The model under review builds one solid part; all positions refer to its coordinate system, in mm. A direction names the side the tool comes from. Round coordinates to 2 decimals unless told otherwise and drop trailing zeros. Order: outer loops, then holes, each group sorted by start corner. A loop starts at its lowest first (then second) coordinate and runs counter-clockwise, first axis right, second up. Notation, with made-up numbers: M 77.5,4 L 134.5,4 A8 ccw 134.5,12 Z; hole C 11,41 d4. An arc over 180 degrees is marked long. Answer as a JSON object with one key per item and string values. Group by question number.
1) The part is to be moulded in two halves that separate along X. For faces 5 (the cylindrical face through (58, 1.61, -96.59)), 6 (the flat face through (-12.7, 2, -57)), 7 (the flat face through (63.5, 2, -95)), 8 (the flat face through (57, 2, -50.8)), say which applies: +X half, -X half, draft (parallel to the pull), parting line (faces both ways), or undercut.
2) Consider section D-D, the plane y = 2.2. Count the separate pieces of the cut face and the enclosed holes in it, then the cut area to 3 significant figures.
3) Consider section B-B, the plane z = -95.25. Write out the cut boundary in (x, y) (1 decimal), then the cut area to 3 significant figures.
4) Insertion check: pin 1 Ø1.6 at (y, z) = (1.5, -77) entering from -X; pin 2 Ø1.6 at (x, y) = (55.5, 1.5) entering from +Z; pin 3 Ø1 at (y, z) = (1.5, -22.5) entering from -X (3 decimals); pin 4 Ø1.9 at (x, z) = (57.15, -95.25) entering from +Y. Each pin has a flat end and moves straight along its axis. Give the tip position at first contact, or say it passes through.
5) Consider section A-A, the plane x = 57.15. Write out the cut boundary in (y, z) (1 decimal).
6) For faces 1 (the flat face through (50.8, 2, -77)), 2 (the flat face through (0, 2, -77)), 3 (the cylindrical face through (2.86, 1.57, -51.71)), 4 (the flat face through (0, 2, -124)), list the 3-axis set-ups (+Z, -Z, +X, -X, +Y, -Y) from which the entire face can be reached by the end or side of a thin tool; tool diameter is ignored.
7) Consider section C-C, the plane z = -57.15. Write out the cut boundary in (x, y) (1 decimal).
8) To check wall thickness, follow line 1 (Z direction, x = 57.15, y = 2.25); line 2 (X direction, y = 1.2, z = -95.25); line 3 (Z direction, x = 53.5, y = 1.7). State the ranges of each line that lie inside material, in increasing order.
```python
from build123d import *

# Parameters (mm, degrees)
SKETCH1_W           = 50.8
SKETCH1_H           = 76.2
BOSS_EXTRUDE1_DEPTH = 3.175
SKETCH2_W           = 18.415
SKETCH2_H           = 63.5
CUT_EXTRUDE1_DEPTH  = 3.175
SKETCH3_W           = 12.7
SKETCH3_H           = 12.7
SKETCH3_R           = 1.5875
BOSS_EXTRUDE2_DEPTH = 3.175
SKETCH7_W           = 50.8
SKETCH7_H           = 12.7
BOSS_EXTRUDE3_DEPTH = 3.175
SKETCH8_W           = 50.8
SKETCH8_H           = 57.15
BOSS_EXTRUDE4_DEPTH = 3.175
LPATTERN1_COUNT     = 2
LPATTERN1_PITCH     = 38.1
FILLET1_R           = 8.89
SKETCH9_W           = 6.35
SKETCH9_H           = 6.35
CUT_EXTRUDE2_DEPTH  = 3.175
SKETCH10_W          = 3.81
SKETCH10_H          = 50.8
CUT_EXTRUDE3_DEPTH  = 3.175
FILLET2_R           = 3.175
FILLET3_R           = 1.27


with BuildPart() as part:
    # Sketch1 → Boss-Extrude1 (new body)
    with BuildSketch(Plane(origin=(0, 0, 0), x_dir=(1, 0, 0), z_dir=(0, 1, 0))):
        with Locations((25.4, 38.1)):
            Rectangle(SKETCH1_W, SKETCH1_H)
    extrude(amount=BOSS_EXTRUDE1_DEPTH)

    # Sketch2 → Cut-Extrude1 (cut)
    with BuildSketch(Plane(origin=(0, 3.175, 0), x_dir=(1, 0, 0), z_dir=(0, 1, 0))):
        with Locations((13.0175, 31.75)):
            Rectangle(SKETCH2_W, SKETCH2_H)
        with Locations((37.7825, 31.75)):
            Rectangle(SKETCH2_W, SKETCH2_H)
    extrude(amount=-CUT_EXTRUDE1_DEPTH, mode=Mode.SUBTRACT)

    # Sketch3 → Boss-Extrude2 (add)
    with BuildSketch(Plane(origin=(0, 3.175, 0), x_dir=(1, 0, 0), z_dir=(0, 1, 0))):
        with Locations((-6.35, 57.15)):
            Rectangle(SKETCH3_W, SKETCH3_H)
        with Locations((-6.35, 57.15)):
            Circle(SKETCH3_R, mode=Mode.SUBTRACT)
        with Locations((57.15, 57.15)):
            Rectangle(SKETCH3_W, SKETCH3_H)
        with Locations((57.15, 57.15)):
            Circle(SKETCH3_R, mode=Mode.SUBTRACT)
    boss_extrude2 = extrude(amount=-BOSS_EXTRUDE2_DEPTH)

    # Sketch7 → Boss-Extrude3 (add)
    with BuildSketch(Plane(origin=(0, 3.175, 0), x_dir=(1, 0, 0), z_dir=(0, 1, 0))):
        with Locations((25.4, 82.55)):
            Rectangle(SKETCH7_W, SKETCH7_H)
    extrude(amount=-BOSS_EXTRUDE3_DEPTH)

    # Sketch8 → Boss-Extrude4 (add)
    with BuildSketch(Plane.XZ):
        with Locations((25.4, -117.475)):
            Rectangle(SKETCH8_W, SKETCH8_H)
    extrude(amount=-BOSS_EXTRUDE4_DEPTH)

    # LPattern1: Boss-Extrude2 ×2
    with Locations(*[(0, 0, -i * LPATTERN1_PITCH) for i in range(1, LPATTERN1_COUNT)]):
        add(boss_extrude2)

    # Fillet1
    fillet1_edges = [part.edges().sort_by_distance(p)[0] for p in [
        (3.81, 1.5875, -63.5),
        (22.225, 1.5875, -63.5),
        (28.575, 1.5875, -63.5),
        (46.99, 1.5875, -63.5),
    ]]
    fillet(fillet1_edges, radius=FILLET1_R)

    # Sketch9 → Cut-Extrude2 (cut)
    with BuildSketch(Plane(origin=(0, 3.175, 0), x_dir=(1, 0, 0), z_dir=(0, 1, 0))):
        with Locations((25.4, 3.175)):
            Rectangle(SKETCH9_W, SKETCH9_H)
    extrude(amount=-CUT_EXTRUDE2_DEPTH, mode=Mode.SUBTRACT)

    # Sketch10 → Cut-Extrude3 (cut)
    with BuildSketch(Plane(origin=(0, 3.175, 0), x_dir=(1, 0, 0), z_dir=(0, 1, 0))):
        with Locations((1.905, 25.4)):
            Rectangle(SKETCH10_W, SKETCH10_H)
        with Locations((48.895, 25.4)):
            Rectangle(SKETCH10_W, SKETCH10_H)
    extrude(amount=-CUT_EXTRUDE3_DEPTH, mode=Mode.SUBTRACT)

    # Fillet2
    fillet2_edges = [part.edges().sort_by_distance(p)[0] for p in [
        (3.81, 1.5875, -50.8),
        (46.99, 1.5875, -50.8),
    ]]
    fillet(fillet2_edges, radius=FILLET2_R)

    # Fillet3
    fillet3_edges = [part.edges().sort_by_distance(p)[0] for p in [
        (0, 1.5875, -63.5),
        (50.8, 1.5875, -63.5),
    ]]
    fillet(fillet3_edges, radius=FILLET3_R)


solid = part.part
```
Results list:
{
 "1": {"face 5": "undercut", "face 6": "-X half", "face 7": "+X half", "face 8": "draft"},
 "2": {"separate pieces": "1", "enclosed holes": "4", "area": "5,330 mm^2"},
 "3": {"outline": "M -12.7,0 L -7.9,0 L -7.9,3.2 L -12.7,3.2 Z; M -4.8,0 L 55.6,0 L 55.6,3.2 L -4.8,3.2 Z; M 58.7,0 L 63.5,0 L 63.5,3.2 L 58.7,3.2 Z", "area": "222 mm^2"},
 "4": {"pin 1": "x = 0", "pin 2": "z = -50.8", "pin 3": "x = 22.225", "pin 4": "through"},
 "5": {"outline": "M 0,-101.6 L 3.2,-101.6 L 3.2,-96.8 L 0,-96.8 Z; M 0,-93.7 L 3.2,-93.7 L 3.2,-88.9 L 0,-88.9 Z; M 0,-63.5 L 3.2,-63.5 L 3.2,-58.7 L 0,-58.7 Z; M 0,-55.6 L 3.2,-55.6 L 3.2,-50.8 L 0,-50.8 Z"},
 "6": {"face 1": "+X, +Y, -Y", "face 2": "-X, +Y, -Y", "face 3": "+Z, +Y, -Y", "face 4": "-Z, -X, +Y, -Y"},
 "7": {"outline": "M -12.7,0 L -7.9,0 L -7.9,3.2 L -12.7,3.2 Z; M -4.8,0 L 4.2,0 L 4.2,3.2 L -4.8,3.2 Z; M 21.9,0 L 28.9,0 L 28.9,3.2 L 21.9,3.2 Z; M 46.6,0 L 55.6,0 L 55.6,3.2 L 46.6,3.2 Z; M 58.7,0 L 63.5,0 L 63.5,3.2 L 58.7,3.2 Z"},
 "8": {"line 1": "-101.6 to -96.84, -93.66 to -88.9, -63.5 to -58.74, -55.56 to -50.8", "line 2": "-12.7 to -7.94, -4.76 to 55.56, 58.74 to 63.5", "line 3": "-101.6 to -88.9, -63.5 to -50.8"}
}
